Verification items for the finished model (mm, model axes). Face numbers are marked on the shaded views. A direction names the side the tool comes from. Round coordinates to 2 decimals unless told otherwise and drop trailing zeros. Write each loop counter-clockwise with the first axis right and the second up, starting at its lowest first coordinate (ties: lowest second). Pieces come first, ordered by that corner, then holes. Notation, with made-up numbers: (-2.75, -16) -> (55.25, -16) arc R22 ccw to (55.25, 6) -> close; hole circle Ø9 at (-24.75, 83.25). An arc over 180 degrees is marked (long way). Answer as a JSON object with one key per item and string values. Group by question number.
(1) Gauge pin test, flat ends, axial feed: pin 1 Ø4.5 at (x, y) = (7.5, 16) entering from -Z; pin 2 Ø1.2 at (y, z) = (47, -4) entering from +X; pin 3 Ø1.8 at (x, y) = (6.95, 16.88) entering from -Z; pin 4 Ø1.5 at (y, z) = (-2, -4.5) entering from -X. Record the tip position at first contact, or that the pin passes through.
(2) Draft check along Y on the marked faces 1, 2 and 3. Enter one of: released by +Y, released by -Y, zero draft, split by the parting line, or undercut.
(3) Sectioned sample at D-D on z = 2.75. Record the cut outline in (x, y), and give its area (3 significant figures).
(4) Sectioned sample at A-A on z = -9.75. Record the cut outline in (x, y), and give its area (3 significant figures).
(5) Sectioned sample at B-B on z = -3.75. Count the separate pieces of the cut face and the enclosed holes in it, and give its area (3 significant figures).
(6) Set-up check for the marked faces 4, 5 and 6: record each of +Z, -Z, +X, -X, +Y, -Y from which the full face is reachable in a straight line by a thin tool's end or side.
(7) Sectioned sample at C-C on x = 16. Record the cut outline in (y, z), and give its area (4 significant figures).
(8) Scan lines: L1, parallel to X at y = 49.4, z = -3.75 (3 decimals); L2, parallel to Z at x = 24.85, y = 50.2 (3 decimals); L3, parallel to Y at x = 27.5, z = -1.25. Record each from-to range of solid material in increasing order. Write a range as from..to.
```python
from build123d import *

# Parameters (mm, degrees)
BOSS_EXTRUDE1_DEPTH = 4
SKETCH2_R           = 1.5
BOSS_EXTRUDE2_DEPTH = 2
BOSS_EXTRUDE3_DEPTH = 5.5
SKETCH4_R           = 2.125
BOSS_EXTRUDE4_DEPTH = 3
SKETCH6_W           = 31
SKETCH6_H           = 15.5
SKETCH6_R           = 2.155122413
SKETCH6_R_2         = 2.125
BOSS_EXTRUDE5_DEPTH = 5.5
CUT_EXTRUDE4_DEPTH  = 3


with BuildPart() as part:
    # Sketch1 → Boss-Extrude1 (new body)
    with BuildSketch(Plane.XY):
        Polygon((0, 51), (31, 51), (31, 36.5), (27, 36.5), (27, 0), (0, 0), align=None)
        Polygon((24.165093822, 18.975641236), (21.740222692, 18.975641236), (20.527787127, 16.875641236), (21.740222692, 14.775641236), (24.165093822, 14.775641236), (25.377529388, 16.875641236), align=None, mode=Mode.SUBTRACT)
        Polygon((24.165093822, 10.975641236), (21.740222692, 10.975641236), (20.527787127, 8.875641236), (21.740222692, 6.775641236), (24.165093822, 6.775641236), (25.377529388, 8.875641236), align=None, mode=Mode.SUBTRACT)
        Polygon((8.165093822, 18.975641236), (5.740222692, 18.975641236), (4.527787127, 16.875641236), (5.740222692, 14.775641236), (8.165093822, 14.775641236), (9.377529388, 16.875641236), align=None, mode=Mode.SUBTRACT)
        Polygon((8.165093822, 10.975641236), (5.740222692, 10.975641236), (4.527787127, 8.875641236), (5.740222692, 6.775641236), (8.165093822, 6.775641236), (9.377529388, 8.875641236), align=None, mode=Mode.SUBTRACT)
    extrude(amount=BOSS_EXTRUDE1_DEPTH)

    # Sketch2 → Boss-Extrude2 (add)
    with BuildSketch(Plane.XY.offset(4)):
        Polygon((0, 51), (31, 51), (31, 36.5), (27, 36.5), (27, -2), (0, -2), align=None)
        with Locations((22.952658257, 16.875641236)):
            Circle(SKETCH2_R, mode=Mode.SUBTRACT)
        with Locations((22.952658257, 8.875641236)):
            Circle(SKETCH2_R, mode=Mode.SUBTRACT)
        with Locations((6.952658257, 8.875641236)):
            Circle(SKETCH2_R, mode=Mode.SUBTRACT)
        with Locations((6.952658257, 16.875641236)):
            Circle(SKETCH2_R, mode=Mode.SUBTRACT)
    extrude(amount=-BOSS_EXTRUDE2_DEPTH)

    # Sketch3 → Boss-Extrude3 (add)
    with BuildSketch(Plane(origin=(0, 51, 0), x_dir=(1, 0, 0), z_dir=(0, 1, 0))):
        Polygon((10.9, 0), (20.3, 0), (21.8, 1.5), (21.8, 6.25), (31, 6.25), (31, 11.5), (0, 11.5), (0, 11.25), (0, 6.25), (1.8, 6.25), (9.4, 6.25), (9.4, 1.5), align=None)
    extrude(amount=-BOSS_EXTRUDE3_DEPTH)

    # Sketch4 → Boss-Extrude4 (add)
    with BuildSketch(Plane(origin=(0, 51, 0), x_dir=(1, 0, 0), z_dir=(0, 1, 0))):
        Polygon((31, -4), (0, -4), (0, 11.5), (31, 11.5), (31, 0), align=None)
        with Locations((6.35, 3.75)):
            Circle(SKETCH4_R, mode=Mode.SUBTRACT)
        with Locations((24.85, 3.75)):
            Circle(SKETCH4_R, mode=Mode.SUBTRACT)
    extrude(amount=-BOSS_EXTRUDE4_DEPTH)

    # Sketch6 → Boss-Extrude5 (add)
    with BuildSketch(Plane.XZ):
        with Locations((15.5, -3.75)):
            Rectangle(SKETCH6_W, SKETCH6_H)
        with Locations((6.35, -3.75)):
            Circle(SKETCH6_R, mode=Mode.SUBTRACT)
        with Locations((24.85, -3.75)):
            Circle(SKETCH6_R_2, mode=Mode.SUBTRACT)
    extrude(amount=BOSS_EXTRUDE5_DEPTH)

    # Sketch7 → Cut-Extrude4 (cut)
    with BuildSketch(Plane.XZ):
        Polygon((10.9, 0), (0, 0), (0, -6.25), (9.4, -6.25), (9.4, -1.5), align=None)
        Polygon((20.3, 0), (31, 0), (31, -6.25), (21.8, -6.25), (21.8, -1.5), align=None)
    extrude(amount=CUT_EXTRUDE4_DEPTH, mode=Mode.SUBTRACT)


solid = part.part
```
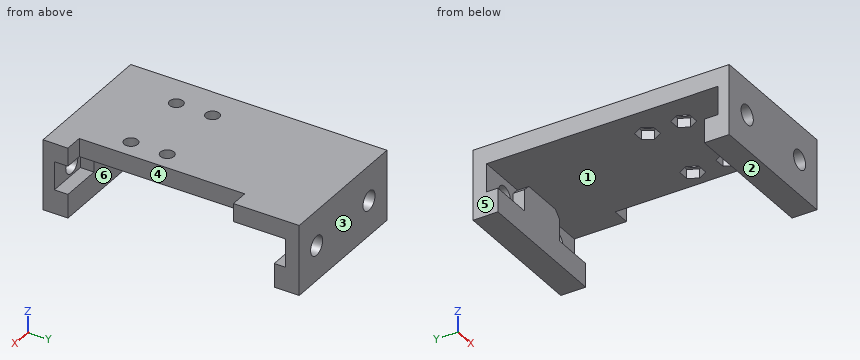
Computed values:
{
 "1": {"pin 1": "z = 0", "pin 2": "x = 21.8", "pin 3": "through", "pin 4": "x = 9.4"},
 "2": {"face 1": "undercut", "face 2": "zero draft", "face 3": "released by +Y"},
 "3": {"outline": "(0, -5.5) -> (31, -5.5) -> (31, 0) -> (27, 0) -> (27, 36.5) -> (31, 36.5) -> (31, 51) -> (0, 51) -> close; hole circle Ø3 at (6.95, 8.88); hole circle Ø3 at (6.95, 16.88); hole circle Ø3 at (22.95, 8.88); hole circle Ø3 at (22.95, 16.88)", "area": "1,580 mm2"},
 "4": {"outline": "(0, -5.5) -> (31, -5.5) -> (31, 0) -> (0, 0) -> close; (0, 45.5) -> (31, 45.5) -> (31, 51) -> (0, 51) -> close", "area": "341 mm2"},
 "5": {"separate pieces": "6", "enclosed holes": "0", "area": "192 mm2"},
 "6": {"face 4": "+Z, -Z, +X", "face 5": "+Z, -Z, -X, +Y, -Y", "face 6": "-Z, +X, -X"},
 "7": {"outline": "(-5.5, -11.5) -> (0, -11.5) -> (0, 0) -> (45.5, 0) -> (45.5, -11.5) -> (51, -11.5) -> (51, 4) -> (-5.5, 4) -> close", "area": "352.5 mm2"},
 "8": {"L1": "0..4.225, 8.475..22.725, 26.975..31", "L2": "-11.5..-5.875, -1.625..4", "L3": "-5.5..-3, 48..51"}
}
